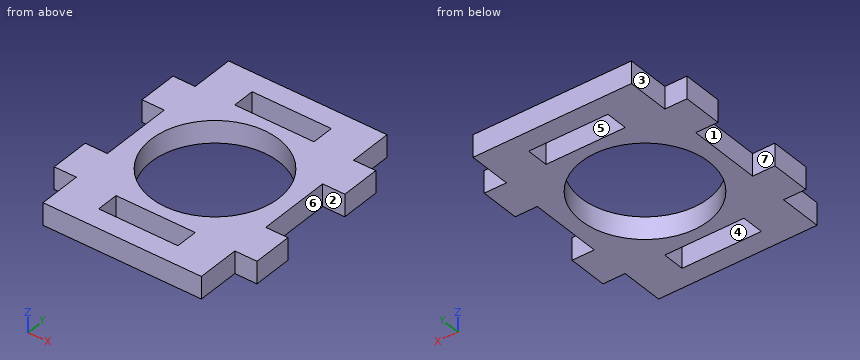
```python
from build123d import *

# Parameters (mm, degrees)
SKETCH_1_R      = 8.05
SKETCH_1_W      = 10
SKETCH_1_H      = 2.8
EXTRUDE_1_DEPTH = 1.4


with BuildPart() as part:
    # Эскиз1 → Бобышка-Вытянуть1 (new, symmetric)
    with BuildSketch(Plane.XY):
        Polygon((-10, 9.6), (-12.8, 9.6), (-12.8, 4.6), (-10, 4.6), (-10, -4.6), (-12.8, -4.6), (-12.8, -9.6), (-10, -9.6), (-10, -15), (10, -15), (10, -9.6), (12.8, -9.6), (12.8, -4.6), (10, -4.6), (10, 4.6), (12.8, 4.6), (12.8, 9.6), (10, 9.6), (10, 15), (-10, 15), align=None)
        Circle(SKETCH_1_R, mode=Mode.SUBTRACT)
        with Locations((0, -11)):
            Rectangle(SKETCH_1_W, SKETCH_1_H, mode=Mode.SUBTRACT)
        with Locations((0, 11)):
            Rectangle(SKETCH_1_W, SKETCH_1_H, mode=Mode.SUBTRACT)
    extrude(amount=EXTRUDE_1_DEPTH, both=True)


solid = part.part
```
The listing builds one solid part. Answer for the finished solid, in the listing's coordinates (mm). Face numbers are marked on the shaded views. A direction names the side the tool comes from. Round coordinates to 2 decimals unless told otherwise and drop trailing zeros. Order: outer loops, then holes, each group sorted by start corner. A loop starts at its lowest first (then second) coordinate and runs counter-clockwise, first axis right, second up. Notation, with made-up numbers: (-11, -28.75) -> (0, -28.75) arc R35 ccw to (0, 4.25) -> close; hole circle Ø8 at (76, 36.25). An arc over 180 degrees is marked (long way). Answer as CSV lines item,"result". Start each with the question number.
(1) For a pull along X with two mould halves and no side action, classify the marked faces 4, 5, 6 and 7 as +X half, -X half, draft (parallel to the pull), parting line (faces both ways), or undercut.
(2) The part is cut by section C-C (y = -12). Determine the outline of the cut face in (x, z).
(3) The part is cut by section A-A (x = 11). Determine the outline of the cut face in (y, z), then the cut area to 3 significant figures.
(4) Find the intervals of material crossed by probe 1 along Y at (x, z) = (0, 0.45); probe 2 along Y at (x, z) = (3, 0.4); probe 3 along X at (y, z) = (6.5, 0.5), in increasing order. Write a range as from..to.
(5) The part is cut by section D-D (z = -0.6). Count the separate pieces of the cut face and the enclosed holes in it, then the cut area to 3 significant figures.
(6) The part is cut by section B-B (x = 0). Determine the outline of the cut face in (y, z), then the cut area to 3 significant figures.
(7) A tool of negligible diameter and unlimited length cuts with its end or side. For the marked faces 1, 2 and 3, from which of +Z, -Z, +X, -X, +Y, -Y can it reach the whole face along a straight path? Write none if from no direction.
(8) Flat-ended cylindrical pins translate along their axes: pin 1 Ø1.5 at (y, z) = (-10.5, 0) entering from +X; pin 2 Ø13 at (x, y) = (0, 0) entering from +Z; pin 3 Ø0.8 at (y, z) = (13.5, 0) entering from -X; pin 4 Ø1.4 at (x, z) = (-11, 0) entering from +Y. Find the tip coordinate at first contact, or state that the pin passes through.
Evaluation:
1,face 4,"undercut"
1,face 5,"undercut"
1,face 6,"+X half"
1,face 7,"draft"
2,outline,"(-10, -1.4) -> (-5, -1.4) -> (-5, 1.4) -> (-10, 1.4) -> close; (5, -1.4) -> (10, -1.4) -> (10, 1.4) -> (5, 1.4) -> close"
3,outline,"(-9.6, -1.4) -> (-4.6, -1.4) -> (-4.6, 1.4) -> (-9.6, 1.4) -> close; (4.6, -1.4) -> (9.6, -1.4) -> (9.6, 1.4) -> (4.6, 1.4) -> close"
3,area,"28.0 mm²"
4,probe 1,"-15..-12.4, -9.6..-8.05, 8.05..9.6, 12.4..15"
4,probe 2,"-15..-12.4, -9.6..-7.47, 7.47..9.6, 12.4..15"
4,probe 3,"-12.8..-4.75, 4.75..12.8"
5,separate pieces,"1"
5,enclosed holes,"3"
5,area,"396 mm²"
6,outline,"(-15, -1.4) -> (-12.4, -1.4) -> (-12.4, 1.4) -> (-15, 1.4) -> close; (-9.6, -1.4) -> (-8.05, -1.4) -> (-8.05, 1.4) -> (-9.6, 1.4) -> close; (8.05, -1.4) -> (9.6, -1.4) -> (9.6, 1.4) -> (8.05, 1.4) -> close; (12.4, -1.4) -> (15, -1.4) -> (15, 1.4) -> (12.4, 1.4) -> close"
6,area,"23.2 mm²"
7,face 1,"+Z, -Z, -X"
7,face 2,"+Z, -Z, +X"
7,face 3,"+Z, -Z, -X, +Y"
8,pin 1,"x = 10"
8,pin 2,"through"
8,pin 3,"x = -10"
8,pin 4,"y = 9.6"
